Source: CAD feature listing. Evaluate the final solid. Frame: model axes, mm. Coordinates: 2 decimals unless noted, no trailing zeros. Write each loop counter-clockwise with the first axis right and the second up, starting at its lowest first coordinate (ties: lowest second). Pieces come first, ordered by that corner, then holes. Notation, with made-up numbers: M -33.5,77 L -16.5,77 A16 ccw -16.5,104 Z; hole C 79,-23.5 d7. An arc over 180 degrees is marked long. One line per item, written item: value. Start each with the question number.
Item 1: Cut plane D-D, the plane y = -10.5. Output: boundary loops of the cut face in (x, z).
Item 2: Pin query (flat end, axial travel): P1, Ø4, axis at y = 3.5, z = 17, coming from the +X side; P2, Ø1, axis at y = 9.5, z = 7, coming from the +X side; P3, Ø5, axis at x = 8, z = 16.5, coming from the -Y side; P4, Ø1.5, axis at y = 4.5, z = 7, coming from the -X side. Return the tip coordinate at first contact, or that it passes through.
Item 3: Cut plane C-C, the plane x = -5. Output: boundary loops of the cut face in (y, z), then the cut area to 3 significant figures.
Item 4: Cut plane A-A, the plane z = 21.75. Output: boundary loops of the cut face in (x, y).
Item 5: Ray query, L1, parallel to X at y = 2.75, z = 8; L2, parallel to Y at x = -1.75, z = 3.25. Return the intervals inside material, ascending. Write a range as from..to.
Item 6: Cut plane B-B, the plane y = 4. Output: boundary loops of the cut face in (x, z), then the cut area to 3 significant figures.
```python
from build123d import *

# Parameters (mm, degrees)
F1_DEPTH = 25.4


with BuildPart() as f1:
    # F0 (on Top) → F1 (new body)
    with BuildSketch(Plane.XY):
        with BuildLine():
            ThreePointArc((0, -6.35), (-6.35, 0), (0, 6.35))
            Line((0, 6.35), (0, 12.7))
            Line((0, 12.7), (-6.35, 12.7))
            Line((-6.35, 12.7), (-13.716, 0))
            Line((-13.716, 0), (-6.35, -12.7))
            Line((-6.35, -12.7), (0, -12.7))
            Line((0, -12.7), (0, -6.35))
        make_face()
        with BuildLine():
            Line((0, 12.7), (0, 6.35))
            ThreePointArc((0, 6.35), (4.490128, 4.490128), (6.35, 0))
            ThreePointArc((6.35, 0), (4.490128, -4.490128), (0, -6.35))
            Line((0, -6.35), (0, -12.7))
            Line((0, -12.7), (6.35, -12.7))
            Line((6.35, -12.7), (13.716, 0))
            Line((13.716, 0), (6.35, 12.7))
            Line((6.35, 12.7), (0, 12.7))
        make_face()
    extrude(amount=F1_DEPTH)


solid = f1.part
```
From the geometry:
1. outline: M -7.63,0 L 7.63,0 L 7.63,25.4 L -7.63,25.4 Z
2. P1: stops at x = 12.85
2. P2: stops at x = 8.5
2. P3: stops at y = -12.7
2. P4: stops at x = -11.54
3. outline: M -12.7,0 L -3.91,0 L -3.91,25.4 L -12.7,25.4 Z; M 3.91,0 L 12.7,0 L 12.7,25.4 L 3.91,25.4 Z
3. area: 446 mm²
4. outline: M -13.72,0 L -6.35,-12.7 L 6.35,-12.7 L 13.72,0 L 6.35,12.7 L -6.35,12.7 Z; hole C 0,0 d12.7
5. L1: x = -12.12..-5.72, 5.72..12.12
5. L2: y = -12.7..-6.1, 6.1..12.7
6. outline: M -11.4,0 L -4.93,0 L -4.93,25.4 L -11.4,25.4 Z; M 4.93,0 L 11.4,0 L 11.4,25.4 L 4.93,25.4 Z
6. area: 328 mm²
